Input: part model. Units: mm. Frame: model coordinates. Coordinates: 2 decimals unless noted, no trailing zeros. Loops run counter-clockwise (first coordinate to the right, second up) from the corner with the lowest first, then second, coordinate; pieces in that order, holes last.
Item 1: Pull-direction query (X, two-part tool) for faces 1 (the flat face through (29.741, -1.565, -9.664)), 2 (the cylindrical face through (-57.095, -1.565, 2.513)); classes: released by +X, released by -X, zero draft, split by the parting line, or undercut.
Item 2: Section C-C on y = -2. Give the number of separate pieces and of enclosed holes in the cut face, and give its area (3 significant figures).
Item 3: Section A-A on z = -12. Return loops of the section in (x, y) (3 decimals), and give its area (3 significant figures).
Item 4: Ray query, line 1 along X through (y, z) = (-1.85, -38); line 2 along X through (y, z) = (-2.4, 27); line 3 along X through (y, z) = (-1.1, -18). Return the intervals inside material, ascending.
Item 5: Contact query for flat-ended pins moving along their axis: P1, Ø1.5, axis at x = -26.5, y = -2.5, coming from the +Z side; P2, Ø1, axis at y = -1.5, z = -1.5, coming from the +X side. Output: stop coordinate, or through.
Item 6: Section B-B on z = -47. Return loops of the section in (x, y) (3 decimals), and give its area (3 significant figures).
```python
from build123d import *

# Parameters (mm, degrees)
F0_R     = 57.15
F0_R_2   = 1.5875
F1_DEPTH = 3.175


with BuildPart() as f1:
    # F0 (on Front) → F1 (new body)
    with BuildSketch(Plane.XZ):
        Circle(F0_R)
        with BuildLine():
            ThreePointArc((0, -53.161082), (-9.231325, -52.353446), (-18.182161, -49.955077))
            Line((-18.182161, -49.955077), (-3.415888, -9.385075))
            ThreePointArc((-3.415888, -9.385075), (-1.734292, -9.835657), (0, -9.987388))
            Line((0, -9.987388), (0, -53.161082))
        make_face(mode=Mode.SUBTRACT)
        with BuildLine():
            ThreePointArc((-50.559194, -16.427678), (-52.643722, -7.398593), (-53.128698, 1.855295))
            Line((-53.128698, 1.855295), (-9.981304, 0.348555))
            ThreePointArc((-9.981304, 0.348555), (-9.890191, -1.389976), (-9.49857, -3.086273))
            Line((-9.49857, -3.086273), (-50.559194, -16.427678))
        make_face(mode=Mode.SUBTRACT)
        with BuildLine():
            ThreePointArc((-31.2473, -43.008219), (-38.240882, -36.928791), (-44.072535, -29.7273))
            Line((-44.072535, -29.7273), (-8.27992, -5.584876))
            ThreePointArc((-8.27992, -5.584876), (-7.184326, -6.937823), (-5.870439, -8.079966))
            Line((-5.870439, -8.079966), (-31.2473, -43.008219))
        make_face(mode=Mode.SUBTRACT)
        with BuildLine():
            ThreePointArc((31.2473, -43.008219), (23.304285, -47.780864), (14.65318, -51.101712))
            Line((14.65318, -51.101712), (2.752897, -9.600493))
            ThreePointArc((2.752897, -9.600493), (4.378183, -8.976605), (5.870439, -8.079966))
            Line((5.870439, -8.079966), (31.2473, -43.008219))
        make_face(mode=Mode.SUBTRACT)
        with BuildLine():
            ThreePointArc((50.559194, -16.427678), (46.93845, -24.957616), (41.891505, -32.72923))
            Line((41.891505, -32.72923), (7.870169, -6.14885))
            ThreePointArc((7.870169, -6.14885), (8.81834, -4.688795), (9.49857, -3.086273))
            Line((9.49857, -3.086273), (50.559194, -16.427678))
        make_face(mode=Mode.SUBTRACT)
        with BuildLine():
            ThreePointArc((-50.559194, 16.427678), (-46.93845, 24.957616), (-41.891505, 32.72923))
            Line((-41.891505, 32.72923), (-7.870169, 6.14885))
            ThreePointArc((-7.870169, 6.14885), (-8.81834, 4.688795), (-9.49857, 3.086273))
            Line((-9.49857, 3.086273), (-50.559194, 16.427678))
        make_face(mode=Mode.SUBTRACT)
        with BuildLine():
            ThreePointArc((-31.2473, 43.008219), (-23.304285, 47.780864), (-14.65318, 51.101712))
            Line((-14.65318, 51.101712), (-2.752897, 9.600493))
            ThreePointArc((-2.752897, 9.600493), (-4.378183, 8.976605), (-5.870439, 8.079966))
            Line((-5.870439, 8.079966), (-31.2473, 43.008219))
        make_face(mode=Mode.SUBTRACT)
        Circle(F0_R_2, mode=Mode.SUBTRACT)
        with BuildLine():
            ThreePointArc((31.2473, 43.008219), (38.240882, 36.928791), (44.072535, 29.7273))
            Line((44.072535, 29.7273), (8.27992, 5.584876))
            ThreePointArc((8.27992, 5.584876), (7.184326, 6.937823), (5.870439, 8.079966))
            Line((5.870439, 8.079966), (31.2473, 43.008219))
        make_face(mode=Mode.SUBTRACT)
        with BuildLine():
            ThreePointArc((50.559194, 16.427678), (52.643722, 7.398593), (53.128698, -1.855295))
            Line((53.128698, -1.855295), (9.981304, -0.348555))
            ThreePointArc((9.981304, -0.348555), (9.890191, 1.389976), (9.49857, 3.086273))
            Line((9.49857, 3.086273), (50.559194, 16.427678))
        make_face(mode=Mode.SUBTRACT)
        with BuildLine():
            ThreePointArc((0, 53.161082), (9.231325, 52.353446), (18.182161, 49.955077))
            Line((18.182161, 49.955077), (3.415888, 9.385075))
            ThreePointArc((3.415888, 9.385075), (1.734292, 9.835657), (0, 9.987388))
            Line((0, 9.987388), (0, 53.161082))
        make_face(mode=Mode.SUBTRACT)
    extrude(amount=F1_DEPTH)


solid = f1.part
```
Results found:
1. face 1: undercut
1. face 2: split by the parting line
2. separate pieces: 1
2. enclosed holes: 11
2. area: 5,490 mm2
3. outline: (-55.876, -3.175) - (-51.789, -3.175) - (-51.789, 0) - (-55.876, 0) - close; (-36.932, -3.175) - (-17.791, -3.175) - (-17.791, 0) - (-36.932, 0) - close; (-8.719, -3.175) - (-4.368, -3.175) - (-4.368, 0) - (-8.719, 0) - close; (0, -3.175) - (3.441, -3.175) - (3.441, 0) - (0, 0) - close; (8.719, -3.175) - (15.359, -3.175) - (15.359, 0) - (8.719, 0) - close; (36.932, -3.175) - (55.876, -3.175) - (55.876, 0) - (36.932, 0) - close
3. area: 180 mm2
4. line 1: x = -42.69 to -37.18, -27.61 to -13.83, 0 to 10.9, 27.61 to 42.69
4. line 2: x = -50.37 to -45.79, -34.56 to -19.62, -7.74 to 0, 9.83 to 19.62, 40.03 to 50.37
4. line 3: x = -54.24 to -26.69, -13.08 to -6.55, 0 to 5.16, 13.08 to 23.04, 50.02 to 54.24
5. P1: stops at z = 51.02
5. P2: stops at x = 57.14
6. outline: (-32.513, -3.175) - (-17.107, -3.175) - (-17.107, 0) - (-32.513, 0) - close; (0, -3.175) - (13.477, -3.175) - (13.477, 0) - (0, 0) - close; (24.842, -3.175) - (32.513, -3.175) - (32.513, 0) - (24.842, 0) - close
6. area: 116 mm2
